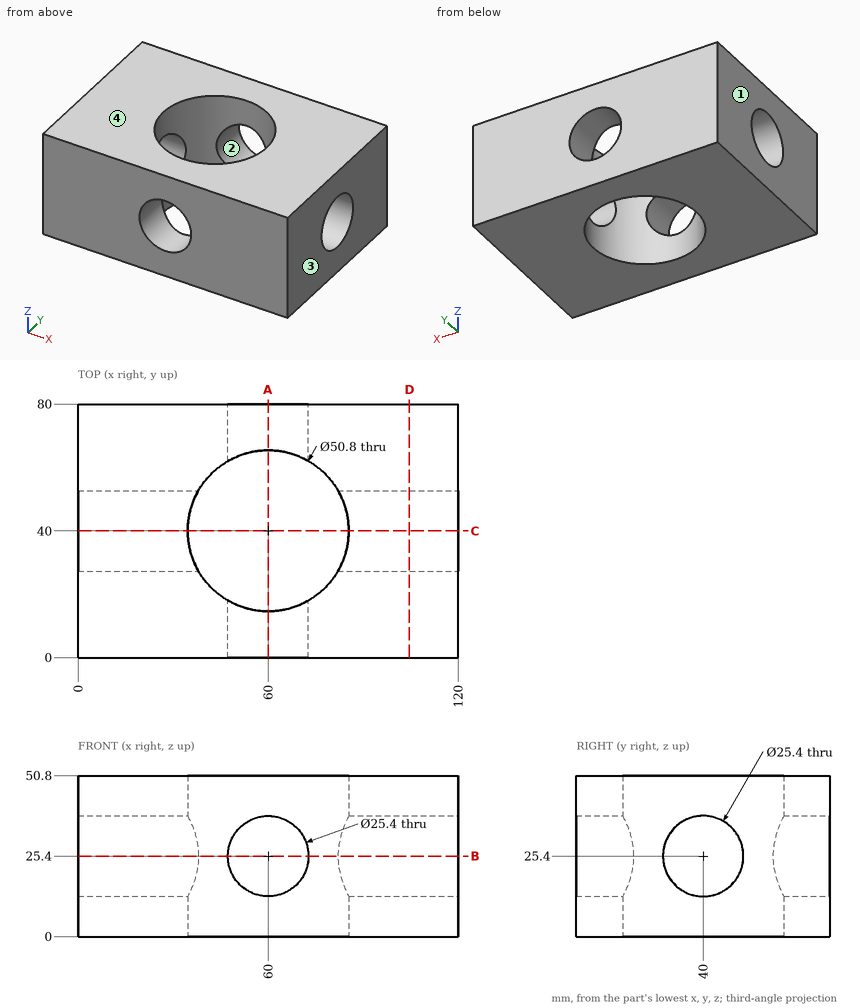
Input: dimensioned drawing with shaded views. Units: mm. Origin: part minimum x, y, z. Coordinates: 2 decimals unless noted, no trailing zeros. Order: outer loops, then holes, each group sorted by start corner. A loop starts at its lowest first (then second) coordinate and runs counter-clockwise, first axis right, second up.
(1) Section query A-A (x = 60). Return the cut outline in (y, z), plus the area to 3 significant figures.
(2) Material intervals for probe 1 along Z at (x, y) = (98, 40); probe 2 along X at (y, z) = (62, 14.5); probe 3 along Y at (x, z) = (82, 16), sorted ascending.
(3) First-contact query: pin 1 (15 mm diameter, centred on x = 60, z = 25.4, fed in from +Y). Flat tip, straight axial feed; report the tip coordinate or a pass-through.
(4) Section query C-C (y = 40). Return the cut outline in (x, z).
(5) Draft query along X for the marked faces 1, 2, 3 and 4. Return one class per face: pulls with the +X half, pulls with the -X half, needs draft (parallel to the pull), parting line crosses it, or undercut.
(6) Section query B-B (z = 25.4). Return the cut outline in (x, y).
(7) Section query D-D (x = 104.5). Return the cut outline in (y, z).
Solution:
1. outline: (0, 0) - (14.6, 0) - (14.6, 12.7) - (0, 12.7) - close; (0, 38.1) - (14.6, 38.1) - (14.6, 50.8) - (0, 50.8) - close; (65.4, 0) - (80, 0) - (80, 12.7) - (65.4, 12.7) - close; (65.4, 38.1) - (80, 38.1) - (80, 50.8) - (65.4, 50.8) - close
1. area: 742 mm2
2. probe 1: z = 0 to 12.7, 38.1 to 50.8
2. probe 2: x = 0 to 47.31, 72.69 to 120
2. probe 3: y = 0 to 27.31, 52.69 to 80
3. pin 1: passes through
4. outline: (0, 0) - (34.6, 0) - (34.6, 12.7) - (0, 12.7) - close; (0, 38.1) - (34.6, 38.1) - (34.6, 50.8) - (0, 50.8) - close; (85.4, 0) - (120, 0) - (120, 12.7) - (85.4, 12.7) - close; (85.4, 38.1) - (120, 38.1) - (120, 50.8) - (85.4, 50.8) - close
5. face 1: pulls with the -X half
5. face 2: undercut
5. face 3: pulls with the +X half
5. face 4: needs draft
6. outline: (0, 0) - (47.3, 0) - (47.3, 18) arc R25.4 cw to (38, 27.3) - (0, 27.3) - close; (0, 52.7) - (38, 52.7) arc R25.4 cw to (47.3, 62) - (47.3, 80) - (0, 80) - close; (72.7, 0) - (120, 0) - (120, 27.3) - (82, 27.3) arc R25.4 cw to (72.7, 18) - close; (72.7, 62) arc R25.4 cw to (82, 52.7) - (120, 52.7) - (120, 80) - (72.7, 80) - close
7. outline: (0, 0) - (80, 0) - (80, 50.8) - (0, 50.8) - close; hole circle Ø25.4 at (40, 25.4)
